For this review, take the finished solid that the model builds, in its own axes (mm). Give positions to 0.01 mm unless a question says otherwise; leave off trailing zeros. Order: outer loops, then holes, each group sorted by start corner. A loop starts at its lowest first (then second) coordinate and runs counter-clockwise, first axis right, second up.
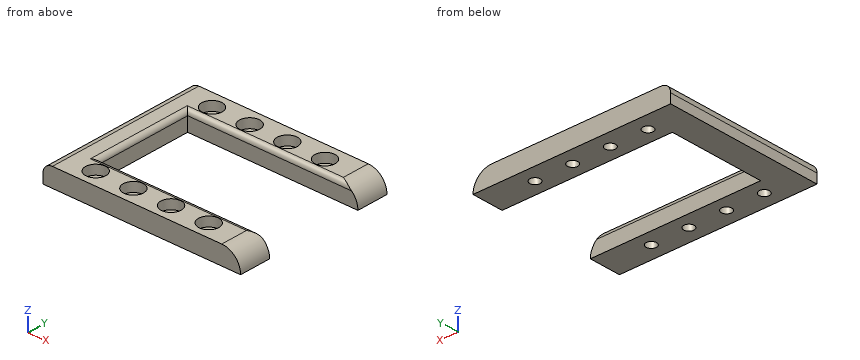
from build123d import *
from OCP.BRepFilletAPI import BRepFilletAPI_MakeFillet

# Parameters (mm, degrees)
SKETCH1_R           = 1.1
BOSS_EXTRUDE1_DEPTH = 4
SKETCH2_W           = 32.7
SKETCH2_H           = 20.5
CUT_EXTRUDE1_DEPTH  = 26.991585177
SKETCH3_R           = 2.15
CUT_EXTRUDE2_DEPTH  = 2
SKETCH6_W           = 4
SKETCH6_H           = 6.75
BOSS_EXTRUDE3_DEPTH = 3.47
FILLET1_R           = 4
FILLET1_R_2         = 2
FILLET1_R_3         = 1


with BuildPart() as part:
    # Sketch1 → Boss-Extrude1 (new body)
    with BuildSketch(Plane.XY):
        with BuildLine():
            Line((19.25, 17), (19.25, 5.6))
            ThreePointArc((19.25, 5.6), (13.65, 0), (19.25, -5.6))
            Line((19.25, -5.6), (19.25, -17))
            Line((19.25, -17), (-19.25, -17))
            Line((-19.25, -17), (-19.25, 17))
            Line((-19.25, 17), (19.25, 17))
        make_face()
        with Locations((12.75, 13.5)):
            Circle(SKETCH1_R, mode=Mode.SUBTRACT)
        with Locations((4.75, 13.5)):
            Circle(SKETCH1_R, mode=Mode.SUBTRACT)
        with Locations((-3.25, 13.5)):
            Circle(SKETCH1_R, mode=Mode.SUBTRACT)
        with Locations((-11.25, 13.5)):
            Circle(SKETCH1_R, mode=Mode.SUBTRACT)
        with Locations(Location((-11.25, -13.5, 0), (0, 0, 180))):
            Circle(SKETCH1_R, mode=Mode.SUBTRACT)
        with Locations(Location((-3.25, -13.5, 0), (0, 0, 180))):
            Circle(SKETCH1_R, mode=Mode.SUBTRACT)
        with Locations(Location((4.75, -13.5, 0), (0, 0, 180))):
            Circle(SKETCH1_R, mode=Mode.SUBTRACT)
        with Locations(Location((12.75, -13.5, 0), (0, 0, 180))):
            Circle(SKETCH1_R, mode=Mode.SUBTRACT)
    extrude(amount=BOSS_EXTRUDE1_DEPTH)

    # Sketch2 → Cut-Extrude1 (cut, through all)
    with BuildSketch(Plane.XY.offset(4)):
        with Locations((2.9, 0)):
            Rectangle(SKETCH2_W, SKETCH2_H)
    extrude(amount=-CUT_EXTRUDE1_DEPTH, mode=Mode.SUBTRACT)

    # Sketch3 → Cut-Extrude2 (cut)
    with BuildSketch(Plane.XY.offset(4)):
        with Locations((12.75, 13.5)):
            Circle(SKETCH3_R)
        with Locations((4.75, 13.5)):
            Circle(SKETCH3_R)
        with Locations((-3.25, 13.5)):
            Circle(SKETCH3_R)
        with Locations((-11.25, 13.5)):
            Circle(SKETCH3_R)
        with Locations((12.75, -13.5)):
            Circle(SKETCH3_R)
        with Locations((4.75, -13.5)):
            Circle(SKETCH3_R)
        with Locations((-3.25, -13.5)):
            Circle(SKETCH3_R)
        with Locations((-11.25, -13.5)):
            Circle(SKETCH3_R)
    extrude(amount=-CUT_EXTRUDE2_DEPTH, mode=Mode.SUBTRACT)

    # Sketch6 → Boss-Extrude3 (add)
    with BuildSketch(Plane(origin=(19.25, 0, 0), x_dir=(0, 0, -1), z_dir=(1, 0, 0))):
        with Locations((-2, -13.625)):
            Rectangle(SKETCH6_W, SKETCH6_H)
        with Locations((-2, 13.625)):
            Rectangle(SKETCH6_W, SKETCH6_H)
    extrude(amount=BOSS_EXTRUDE3_DEPTH)

    # Fillet1
    fillet1_edges_1 = [part.edges().sort_by_distance(p)[0] for p in [
        (22.72, 13.625, 4),
        (22.72, -13.625, 4),
    ]]
    fillet1_edges_2 = [part.edges().sort_by_distance(p)[0] for p in [
        (-19.25, 0, 4),
    ]]
    fillet1_edges_3 = [part.edges().sort_by_distance(p)[0] for p in [
        (4.635, 10.25, 4),
        (4.635, -10.25, 4),
        (-13.45, 0, 4),
    ]]
    fillet1 = BRepFilletAPI_MakeFillet(part.part.solid().wrapped)
    for e in fillet1_edges_1:
        fillet1.Add(FILLET1_R - 0.0001, e.wrapped)
    for e in fillet1_edges_2:
        fillet1.Add(FILLET1_R_2 - 0.0001, e.wrapped)
    for e in fillet1_edges_3:
        fillet1.Add(FILLET1_R_3 - 0.0001, e.wrapped)
    add(Compound.cast(fillet1.Shape()), mode=Mode.REPLACE)  # a hair under: the kernel refuses the full size


solid = part.part
1) We need section C-C on z = 1.15. Count the separate pieces of the cut face and the enclosed holes in it, then the cut area to 3 significant figures.
Answer sheet:
separate pieces: 1
enclosed holes: 8
area: 653 mm2
2) We need section B-B on x = 2. Give the boundary of the cut face in (y, z), then the cut area to 3 significant figures.
Answer sheet:
outline: (-17, 0) - (-10.25, 0) - (-10.25, 3) arc R1 ccw to (-11.25, 4) - (-17, 4) - close; (10.25, 0) - (17, 0) - (17, 4) - (11.25, 4) arc R1 ccw to (10.25, 3) - close
area: 53.6 mm2
3) To check wall thickness, follow line 1 (Y direction, x = 12.75, z = 2.85); line 2 (Y direction, x = -5.5, z = 1.95); line 3 (Y direction, x = 4.75, z = 3.6). State the ranges of each line that lie inside material, in increasing order.
Answer sheet:
line 1: y = -17 to -15.65, -11.35 to -10.25, 10.25 to 11.35, 15.65 to 17
line 2: y = -17 to -10.25, 10.25 to 17
line 3: y = -17 to -15.65, -11.35 to -10.45, 10.45 to 11.35, 15.65 to 17
4) We need section D-D on y = -2.5. Give the boundary of the cut face in (x, z), then the cut area to 3 significant figures.
Answer sheet:
outline: (-19.25, 0) - (-13.45, 0) - (-13.45, 3) arc R1 ccw to (-14.45, 4) - (-17.25, 4) arc R2 ccw to (-19.25, 2) - close
area: 22.1 mm2
5) We need section A-A on x = 12.75. Give the boundary of the cut face in (y, z), then the cut area to 3 significant figures.
Answer sheet:
outline: (-17, 0) - (-14.6, 0) - (-14.6, 2) - (-15.65, 2) - (-15.65, 4) - (-17, 4) - close; (-12.4, 0) - (-10.25, 0) - (-10.25, 3) arc R1 ccw to (-11.25, 4) - (-11.35, 4) - (-11.35, 2) - (-12.4, 2) - close; (10.25, 0) - (12.4, 0) - (12.4, 2) - (11.35, 2) - (11.35, 4) - (11.25, 4) arc R1 ccw to (10.25, 3) - close; (14.6, 0) - (17, 0) - (17, 4) - (15.65, 4) - (15.65, 2) - (14.6, 2) - close
area: 27.6 mm2
6) Clearance check with flat-ended pins moving along their axes: pin 1 (1 mm diameter, centred on x = -11, y = 2.5, fed in from +Z); pin 2 (4 mm diameter, centred on x = 4.75, y = 13.5, fed in from +Z); pin 3 (8 mm diameter, centred on x = 17, y = 6.5, fed in from +Z). State where each tip first meets the part, or that it passes through.
Answer sheet:
pin 1: passes through
pin 2: stops at z = 2
pin 3: stops at z = 3.66
